```python
from build123d import *

# Parameters (mm, degrees)
SKETCH_1_W                 = 47
SKETCH_1_H                 = 79
EXTRUDE_1_DEPTH            = 3
HOLE_WIZARD_M31_AT_2_COUNT = 2
HOLE_WIZARD_M31_AT_2_PITCH = 22
HOLE_WIZARD_M31_AT_3_COUNT = 2
HOLE_WIZARD_M31_AT_3_PITCH = 47
HOLE_WIZARD_M31_AT_4_COUNT = 2
HOLE_WIZARD_M31_AT_4_PITCH = 51.894122981
HOLE_WIZARD_M32_AT_2_COUNT = 2
HOLE_WIZARD_M32_AT_2_PITCH = 37
HOLE_WIZARD_M32_AT_3_COUNT = 2
HOLE_WIZARD_M32_AT_3_PITCH = 69
HOLE_WIZARD_M32_AT_4_COUNT = 2
HOLE_WIZARD_M32_AT_4_PITCH = 78.294316524
FILLET_1_R                 = 3


with BuildPart() as part:
    # Эскиз1 → Бобышка-Вытянуть1 (new body)
    with BuildSketch(Plane.XY):
        Rectangle(SKETCH_1_W, SKETCH_1_H)
    extrude(amount=EXTRUDE_1_DEPTH)

    # Эскиз3 → Зенковка для  винта с потайной головкой с внутренним шестигранником M31 (revolve, cut)
    with BuildSketch(Plane(origin=(-11, 23.5, 3), x_dir=(0, -1, 0), z_dir=(1, 0, 0))):
        Polygon((0, 0), (0, 3), (1.7, 3), (1.7, 1.66), (3.36, 0), align=None)
    hole_wizard_m31 = revolve(axis=Axis((-11, 23.5, 9.35), (0, 0, -1)), mode=Mode.SUBTRACT)

    # Зенковка для  винта с потайной головкой с внутренним шестигранником M31 at 2: Зенковка для  винта с потайной головкой с внутренним шестигранником M31 ×2
    with Locations(*[(i * HOLE_WIZARD_M31_AT_2_PITCH, 0, 0) for i in range(1, HOLE_WIZARD_M31_AT_2_COUNT)]):
        add(hole_wizard_m31, mode=Mode.SUBTRACT)

    # Зенковка для  винта с потайной головкой с внутренним шестигранником M31 at 3: Зенковка для  винта с потайной головкой с внутренним шестигранником M31 ×2
    with Locations(*[(0, -i * HOLE_WIZARD_M31_AT_3_PITCH, 0) for i in range(1, HOLE_WIZARD_M31_AT_3_COUNT)]):
        add(hole_wizard_m31, mode=Mode.SUBTRACT)

    # Зенковка для  винта с потайной головкой с внутренним шестигранником M31 at 4: Зенковка для  винта с потайной головкой с внутренним шестигранником M31 ×2
    with Locations(*[Vector(0.42394010604863086, -0.9056902265584386, 0) * (i * HOLE_WIZARD_M31_AT_4_PITCH) for i in range(1, HOLE_WIZARD_M31_AT_4_COUNT)]):
        add(hole_wizard_m31, mode=Mode.SUBTRACT)

    # Эскиз6 → Зенковка для  винта с потайной головкой с внутренним шестигранником M32 (revolve, cut)
    with BuildSketch(Plane(origin=(18.5, 34.5, 0), x_dir=(0, 1, 0), z_dir=(1, 0, 0))):
        Polygon((0, 0), (0, 3), (1.7, 3), (1.7, 1.66), (3.36, 0), align=None)
    hole_wizard_m32 = revolve(axis=Axis((18.5, 34.5, -6.35), (0, 0, 1)), mode=Mode.SUBTRACT)

    # Зенковка для  винта с потайной головкой с внутренним шестигранником M32 at 2: Зенковка для  винта с потайной головкой с внутренним шестигранником M32 ×2
    with Locations(*[(-i * HOLE_WIZARD_M32_AT_2_PITCH, 0, 0) for i in range(1, HOLE_WIZARD_M32_AT_2_COUNT)]):
        add(hole_wizard_m32, mode=Mode.SUBTRACT)

    # Зенковка для  винта с потайной головкой с внутренним шестигранником M32 at 3: Зенковка для  винта с потайной головкой с внутренним шестигранником M32 ×2
    with Locations(*[(0, -i * HOLE_WIZARD_M32_AT_3_PITCH, 0) for i in range(1, HOLE_WIZARD_M32_AT_3_COUNT)]):
        add(hole_wizard_m32, mode=Mode.SUBTRACT)

    # Зенковка для  винта с потайной головкой с внутренним шестигранником M32 at 4: Зенковка для  винта с потайной головкой с внутренним шестигранником M32 ×2
    with Locations(*[Vector(-0.4725758093633575, -0.8812900228668016, 0) * (i * HOLE_WIZARD_M32_AT_4_PITCH) for i in range(1, HOLE_WIZARD_M32_AT_4_COUNT)]):
        add(hole_wizard_m32, mode=Mode.SUBTRACT)

    # Скругление1
    fillet_1_edges = [part.edges().sort_by_distance(p)[0] for p in [
        (23.5, -39.5, 1.5),
        (-23.5, -39.5, 1.5),
        (-23.5, 39.5, 1.5),
        (23.5, 39.5, 1.5),
    ]]
    fillet(fillet_1_edges, radius=FILLET_1_R)


solid = part.part
```
The listing builds one solid part. Answer for the finished solid, in the listing's coordinates (mm). Give positions to 0.01 mm unless a question says otherwise; leave off trailing zeros. Order: outer loops, then holes, each group sorted by start corner. A loop starts at its lowest first (then second) coordinate and runs counter-clockwise, first axis right, second up. Notation, with made-up numbers: (5.25, -22) - (15.25, -22) arc R30 cw to (15.25, 15) - close; hole circle Ø11 at (14.25, -20.75). An arc over 180 degrees is marked (long way). Use one line per item in the form item = value. Start each with the question number.
(1) A cutting plane is placed at B-B, the plane z = 2.4. State how many separate pieces and enclosed holes the cut face has, then the cut area to 3 significant figures.
(2) A cutting plane is placed at C-C, the plane y = -23.5. Write down the section's boundary in (x, z), then the cut area to 3 significant figures.
(3) Consider line 1 (Y direction, x = 18.5, z = 2.7); line 2 (X direction, y = 23.5, z = 0.55); line 3 (X direction, y = -34.5, z = 2.05). Determine where each line is inside the solid, lowest interval first. Write a range as from..to.
(4) Flat-ended cylindrical pins translate along their axes: pin 1 Ø3 at (x, y) = (-11, -23.5) entering from +Z; pin 2 Ø4 at (x, y) = (11, 23.5) entering from +Z. Find the tip coordinate at first contact, or state that the pin passes through.
(5) The mould has two halves that part along X. Classify faces 1 (the cylindrical face through (-22.64, -38.6, 1.52)), 2 (the cylindrical face through (-18.57, -36.2, 2.32)), 3 (the flat face through (0, -39.5, 1)): released by +X, released by -X, zero draft, split by the parting line, or undercut.
(6) A cutting plane is placed at A-A, the plane x = 18.5. Write down the section's boundary in (y, z).
Ans:
q1.separate_pieces = 1
q1.enclosed_holes = 8
q1.area = 3,570 mm^2
q2.outline = (-23.5, 0) - (-12.7, 0) - (-12.7, 1.34) - (-14.36, 3) - (-23.5, 3) - close; (-9.3, 0) - (9.3, 0) - (9.3, 1.34) - (7.64, 3) - (-7.64, 3) - (-9.3, 1.34) - close; (12.7, 0) - (23.5, 0) - (23.5, 3) - (14.36, 3) - (12.7, 1.34) - close
q2.area = 115 mm^2
q3.line_1 = -39.5..-36.2, -32.8..32.8, 36.2..39.5
q3.line_2 = -23.5..-12.7, -9.3..9.3, 12.7..23.5
q3.line_3 = -23.5..-20.2, -16.8..16.8, 20.2..23.5
q4.pin_1 = through
q4.pin_2 = 1.64
q5.face_1 = released by -X
q5.face_2 = undercut
q5.face_3 = zero draft
q6.outline = (-39.5, 0) - (-37.86, 0) - (-36.2, 1.66) - (-36.2, 3) - (-39.5, 3) - close; (-32.8, 1.66) - (-31.14, 0) - (31.14, 0) - (32.8, 1.66) - (32.8, 3) - (-32.8, 3) - close; (36.2, 1.66) - (37.86, 0) - (39.5, 0) - (39.5, 3) - (36.2, 3) - close
